```python
from build123d import *

# Parameters (mm, degrees)
F1_DEPTH = 10
F2_W     = 21.2
F2_H     = 3
F3_DEPTH = 5.35


with BuildPart() as f1:
    # F0 (on Front) → F1 (new body)
    with BuildSketch(Plane.XZ):
        with BuildLine():
            Line((-10.6, -2.53), (-10.6, -3.07))
            Line((-10.6, -3.07), (-7.8, -5.87))
            Line((-7.8, -5.87), (-7.8, -7.9))
            ThreePointArc((-7.8, -7.9), (-8.23934, -8.96066), (-9.3, -9.4))
            Line((-9.3, -9.4), (9.3, -9.4))
            ThreePointArc((9.3, -9.4), (8.23934, -8.96066), (7.8, -7.9))
            Line((7.8, -7.9), (7.8, -5.87))
            Line((7.8, -5.87), (10.6, -3.07))
            Line((10.6, -3.07), (10.6, -2.53))
            Line((10.6, -2.53), (8.07, 0))
            Line((8.07, 0), (-8.07, 0))
            Line((-8.07, 0), (-10.6, -2.53))
        make_face()
    extrude(amount=F1_DEPTH)


with BuildPart() as f3:
    # F2 (on Front) → F3 (new body)
    with BuildSketch(Plane.XZ):
        with Locations((0, -1.5)):
            Rectangle(F2_W, F2_H)
    extrude(amount=F3_DEPTH)


with BuildPart() as f1_1:
    add(f1.part)

    # F4: cut F3
    add(f3.part, mode=Mode.SUBTRACT)


solid = f1_1.part
```
Verification items for the finished model (mm, model axes). A direction names the side the tool comes from. Give positions to 0.01 mm unless a question says otherwise; leave off trailing zeros. Write each loop counter-clockwise with the first axis right and the second up, starting at its lowest first coordinate (ties: lowest second). Pieces come first, ordered by that corner, then holes. Notation, with made-up numbers: M 43.25,-4 L 59.25,-4 A26 ccw 59.25,10 Z; hole C 88,9 d8. An arc over 180 degrees is marked long. One line per question, with ' | ' between items.
1) Section check D-D on y = -2.5. Enter the section's corners in (x, z), plus the area to 3 significant figures.
Result:
outline: M -10.6,-3.07 L -7.8,-5.87 L -7.8,-7.9 A1.5 cw -9.3,-9.4 L 9.3,-9.4 A1.5 cw 7.8,-7.9 L 7.8,-5.87 L 10.6,-3.07 L 10.6,-3 L -10.6,-3 Z | area: 109 mm2
2) Section check A-A on y = -6. Enter the section's corners in (x, z), plus the area to 3 significant figures.
Result:
outline: M -10.6,-3.07 L -7.8,-5.87 L -7.8,-7.9 A1.5 cw -9.3,-9.4 L 9.3,-9.4 A1.5 cw 7.8,-7.9 L 7.8,-5.87 L 10.6,-3.07 L 10.6,-2.53 L 8.07,0 L -8.07,0 L -10.6,-2.53 Z | area: 166 mm2
3) Thickness scan on line 1 along Y through (x, z) = (-7, -2.25); line 2 along X through (y, z) = (-6.75, -8.75); line 3 along X through (y, z) = (-9, -7). Record the ranges inside material, lowest first. Write a range as [from, to].
Result:
line 1: y = [-10, -5.35] | line 2: x = [-8.06, 8.06] | line 3: x = [-7.8, 7.8]
4) Section check C-C on z = -6.5. Enter the section's corners in (x, y), plus the area to 3 significant figures.
Result:
outline: M -7.8,-10 L 7.8,-10 L 7.8,0 L -7.8,0 Z | area: 156 mm2
5) Gauge pin test, flat ends, axial feed: pin 1 Ø2 at (y, z) = (-6.5, -7) entering from +X; pin 2 Ø3 at (x, y) = (-7.5, -1.5) entering from +Z; pin 3 Ø2 at (y, z) = (-4, -7) entering from -X. Record the tip position at first contact, or that the pin passes through.
Result:
pin 1: stops at x = 7.8 | pin 2: stops at z = -3 | pin 3: stops at x = -7.8
6) Set-up check for faces 4 (the flat face through (0, -10, -5)), 5 (the cylindrical face through (-8.23, -4.93, -8.95)), 6 (the cylindrical face through (8.25, -4.93, -8.97)): record each of +Z, -Z, +X, -X, +Y, -Y from which the full face is reachable in a straight line by a thin tool's end or side.
Result:
face 4: +Z, -Z, +X, -X, -Y | face 5: -X, +Y, -Y | face 6: +X, +Y, -Y
7) Section check B-B on x = -2.5. Enter the section's corners in (y, z).
Result:
outline: M -10,-9.4 L 0,-9.4 L 0,-3 L -5.35,-3 L -5.35,0 L -10,0 Z
8) Mould release check, pull along Z, two halves, no side actions. Record for faces 1 (the flat face through (0, -3, -3)), 2 (the flat face through (9.18, -4.93, -4.49)), 3 (the flat face through (0, -5.35, -1)): released by +Z, released by -Z, zero draft, split by the parting line, or undercut.
Result:
face 1: released by +Z | face 2: undercut | face 3: zero draft
